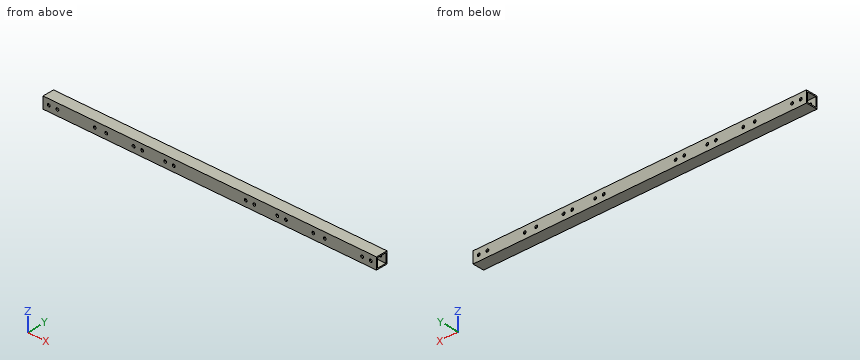
```python
from build123d import *

# Parameters (mm, degrees)
SKETCH1_W           = 20
SKETCH1_H           = 20
SKETCH1_W_2         = 16
SKETCH1_H_2         = 16
BOSS_EXTRUDE1_DEPTH = 580
SKETCH2_R           = 2.5
CUT_EXTRUDE1_DEPTH  = 581.430874437
SKETCH3_R           = 2.5
CUT_EXTRUDE2_DEPTH  = 581.430874437
SKETCH4_R           = 2.5
CUT_EXTRUDE3_DEPTH  = 581.430874437


with BuildPart() as part:
    # Sketch1 → Boss-Extrude1 (new body)
    with BuildSketch(Plane(origin=(0, 0, 0), x_dir=(0, 0, -1), z_dir=(1, 0, 0))):
        Rectangle(SKETCH1_W, SKETCH1_H)
        Rectangle(SKETCH1_W_2, SKETCH1_H_2, mode=Mode.SUBTRACT)
    extrude(amount=BOSS_EXTRUDE1_DEPTH)

    # Sketch2 → Cut-Extrude1 (cut, through all)
    with BuildSketch(Plane(origin=(0, 10, 0), x_dir=(1, 0, 0), z_dir=(0, 1, 0))):
        with Locations(Location((10, 0, 0), (0, 0, 270))):
            Circle(SKETCH2_R)
        with Locations(Location((570, 0, 0), (0, 0, 270))):
            Circle(SKETCH2_R)
        with Locations(Location((25, 0, 0), (0, 0, 270))):
            Circle(SKETCH2_R)
        with Locations(Location((555, 0, 0), (0, 0, 270))):
            Circle(SKETCH2_R)
    extrude(amount=-CUT_EXTRUDE1_DEPTH, mode=Mode.SUBTRACT)

    # Sketch3 → Cut-Extrude2 (cut, through all)
    with BuildSketch(Plane(origin=(0, 10, 0), x_dir=(1, 0, 0), z_dir=(0, 1, 0))):
        with Locations(Location((110, 0, 0), (0, 0, 270))):
            Circle(SKETCH3_R)
        with Locations(Location((90, 0, 0), (0, 0, 270))):
            Circle(SKETCH3_R)
        with Locations(Location((490, 0, 0), (0, 0, 270))):
            Circle(SKETCH3_R)
        with Locations(Location((470, 0, 0), (0, 0, 270))):
            Circle(SKETCH3_R)
    extrude(amount=-CUT_EXTRUDE2_DEPTH, mode=Mode.SUBTRACT)

    # Sketch4 → Cut-Extrude3 (cut, through all)
    with BuildSketch(Plane(origin=(0, 10, 0), x_dir=(1, 0, 0), z_dir=(0, 1, 0))):
        with Locations(Location((157.5, 0, 0), (0, 0, 270))):
            Circle(SKETCH4_R)
        with Locations(Location((172.5, 0, 0), (0, 0, 270))):
            Circle(SKETCH4_R)
        with Locations(Location((212.5, 0, 0), (0, 0, 270))):
            Circle(SKETCH4_R)
        with Locations(Location((227.5, 0, 0), (0, 0, 270))):
            Circle(SKETCH4_R)
        with Locations(Location((352.5, 0, 0), (0, 0, 270))):
            Circle(SKETCH4_R)
        with Locations(Location((367.5, 0, 0), (0, 0, 270))):
            Circle(SKETCH4_R)
        with Locations(Location((407.5, 0, 0), (0, 0, 270))):
            Circle(SKETCH4_R)
        with Locations(Location((422.5, 0, 0), (0, 0, 270))):
            Circle(SKETCH4_R)
    extrude(amount=-CUT_EXTRUDE3_DEPTH, mode=Mode.SUBTRACT)


solid = part.part
```
Here's how the part is built. I have some questions about the finished solid (model axes, mm). Give positions to 0.01 mm unless a question says otherwise; leave off trailing zeros. Write each loop counter-clockwise with the first axis right and the second up, starting at its lowest first coordinate (ties: lowest second). Pieces come first, ordered by that corner, then holes. Notation, with made-up numbers: (12, 44.25) -> (32, 44.25) arc R23 ccw to (32, 58.25) -> close; hole circle Ø4 at (53.5, 26.5). An arc over 180 degrees is marked (long way). Write each question's results on one line, items separated by ' | '.
Item 1: Suppose I cut it at B-B on y = -3.5. Write out the boundary of the cut face in (x, z).
Output:
outline: (0, -10) -> (580, -10) -> (580, -8) -> (0, -8) -> close; (0, 8) -> (580, 8) -> (580, 10) -> (0, 10) -> close
Item 2: If I drill on L1, parallel to Y at x = 232.5, z = 7.75; L2, parallel to Z at x = 212.5, y = -9.2, over which ranges is the centre line in solid material (lowest first)?
Output:
L1: y = -10 to -8, 8 to 10 | L2: z = -10 to -2.5, 2.5 to 10
Item 3: For pin 1 Ø6 at (x, z) = (110, 0) entering from -Y; pin 2 Ø3 at (x, z) = (172.5, 0) entering from +Y, each with a flat end and sliding along its axis, tell me the tip position at first contact or that it passes through.
Output:
pin 1: stops at y = -10 | pin 2: passes through
Item 4: Suppose I cut it at A-A on x = 256. Write out the boundary of the cut face in (y, z), plus the area to 3 significant figures.
Output:
outline: (-10, -10) -> (10, -10) -> (10, 10) -> (-10, 10) -> close; hole (-8, -8) -> (8, -8) -> (8, 8) -> (-8, 8) -> close | area: 144 mm^2
